```python
from build123d import *

# Parameters (mm, degrees)
SKETCH1_W                      = 60
SKETCH1_H                      = 430.5
BASE_FLANGE1_DEPTH             = 4
EDGE_FLANGE1_STRIP_W           = 18
EDGE_FLANGE1_STRIP_H           = 4
EDGE_FLANGE1_STRIP_CUT_DEPTH   = 430.5
EDGE_FLANGE1_DEPTH             = 430.5
EDGE_FLANGE2_STRIP_W           = 18
EDGE_FLANGE2_STRIP_H           = 4
EDGE_FLANGE2_STRIP_CUT_DEPTH   = 55
EDGE_FLANGE2_STRIP_2_W         = 18
EDGE_FLANGE2_STRIP_2_H         = 4
EDGE_FLANGE2_STRIP_CUT_2_DEPTH = 55
EDGE_FLANGE2_STRIP_3_W         = 18
EDGE_FLANGE2_STRIP_3_H         = 4
EDGE_FLANGE2_STRIP_CUT_3_DEPTH = 55
EDGE_FLANGE2_STRIP_4_W         = 18
EDGE_FLANGE2_STRIP_4_H         = 4
EDGE_FLANGE2_STRIP_CUT_4_DEPTH = 55
EDGE_FLANGE2_DEPTH             = 55
EDGE_FLANGE2_BEND_DEPTH        = 55
EDGE_FLANGE2_BEND_2_DEPTH      = 55
EDGE_FLANGE2_BEND_3_DEPTH      = 55
SKETCH18_R                     = 4.6
EXTRUDE1_DEPTH                 = 440.643321341


# Sheet-metal steps are written as plain solids
with BuildPart() as part:
    # Sketch1 → Base-Flange1 (new body)
    with BuildSketch(Plane(origin=(0, 0, 0), x_dir=(1, 0, 0), z_dir=(0, 1, 0))):
        Rectangle(SKETCH1_W, SKETCH1_H)
    extrude(amount=BASE_FLANGE1_DEPTH)

    # Edge-Flange1 strip (across the edge) → Edge-Flange1 strip cut (cut)
    with BuildSketch(Plane(origin=(-30, 4, -215.25), x_dir=(1, 0, 0), z_dir=(0, 0, 1))):
        with Locations((-4, -2)):
            Rectangle(EDGE_FLANGE1_STRIP_W, EDGE_FLANGE1_STRIP_H)
    extrude(amount=EDGE_FLANGE1_STRIP_CUT_DEPTH, mode=Mode.SUBTRACT)

    # Edge-Flange1 section (across the edge) → Edge-Flange1 (add)
    with BuildSketch(Plane(origin=(-30, 4, -215.25), x_dir=(1, 0, 0), z_dir=(0, 0, 1))):
        with BuildLine():
            Line((0, 1), (0, 56))
            Line((0, 56), (4, 56))
            Line((4, 56), (4, 1))
            ThreePointArc((4, 1), (4.292893219, 0.292893219), (5, 0))
            Line((5, 0), (5, -4))
            ThreePointArc((5, -4), (1.464466094, -2.535533906), (0, 1))
        make_face()
    extrude(amount=EDGE_FLANGE1_DEPTH)

    # Edge-Flange2 strip (across the edge) → Edge-Flange2 strip cut (cut)
    with BuildSketch(Plane(origin=(-30, 5, 215.25), x_dir=(0, 0, -1), z_dir=(0, 1, 0))):
        with Locations((-4, -2)):
            Rectangle(EDGE_FLANGE2_STRIP_W, EDGE_FLANGE2_STRIP_H)
    extrude(amount=EDGE_FLANGE2_STRIP_CUT_DEPTH, mode=Mode.SUBTRACT)

    # Edge-Flange2 strip 2 (across the edge) → Edge-Flange2 strip cut 2 (cut)
    with BuildSketch(Plane(origin=(30, 0, 215.25), x_dir=(0, 0, -1), z_dir=(-1, 0, 0))):
        with Locations((-4, -2)):
            Rectangle(EDGE_FLANGE2_STRIP_2_W, EDGE_FLANGE2_STRIP_2_H)
    extrude(amount=EDGE_FLANGE2_STRIP_CUT_2_DEPTH, mode=Mode.SUBTRACT)

    # Edge-Flange2 strip 3 (across the edge) → Edge-Flange2 strip cut 3 (cut)
    with BuildSketch(Plane(origin=(-30, 60, -215.25), x_dir=(0, 0, 1), z_dir=(0, -1, 0))):
        with Locations((-4, -2)):
            Rectangle(EDGE_FLANGE2_STRIP_3_W, EDGE_FLANGE2_STRIP_3_H)
    extrude(amount=EDGE_FLANGE2_STRIP_CUT_3_DEPTH, mode=Mode.SUBTRACT)

    # Edge-Flange2 strip 4 (across the edge) → Edge-Flange2 strip cut 4 (cut)
    with BuildSketch(Plane(origin=(-25, 0, -215.25), x_dir=(0, 0, 1), z_dir=(1, 0, 0))):
        with Locations((-4, -2)):
            Rectangle(EDGE_FLANGE2_STRIP_4_W, EDGE_FLANGE2_STRIP_4_H)
    extrude(amount=EDGE_FLANGE2_STRIP_CUT_4_DEPTH, mode=Mode.SUBTRACT)

    # Edge-Flange2 section (across the edge) → Edge-Flange2 (add)
    with BuildSketch(Plane(origin=(-30, 5, 215.25), x_dir=(0, 0, -1), z_dir=(0, 1, 0))):
        with BuildLine():
            Line((0, 1), (0, 36))
            Line((0, 36), (4, 36))
            Line((4, 36), (4, 1))
            ThreePointArc((4, 1), (4.292893219, 0.292893219), (5, 0))
            Line((5, 0), (5, -4))
            ThreePointArc((5, -4), (1.464466094, -2.535533906), (0, 1))
        make_face()
    extrude(amount=EDGE_FLANGE2_DEPTH)

    # Edge-Flange2 section 2 (across the edge) → Edge-Flange2 bend (add)
    with BuildSketch(Plane(origin=(30, 0, 215.25), x_dir=(0, 0, -1), z_dir=(-1, 0, 0))):
        with BuildLine():
            Line((0, 1), (0, 36))
            Line((0, 36), (4, 36))
            Line((4, 36), (4, 1))
            ThreePointArc((4, 1), (4.292893219, 0.292893219), (5, 0))
            Line((5, 0), (5, -4))
            ThreePointArc((5, -4), (1.464466094, -2.535533906), (0, 1))
        make_face()
    extrude(amount=EDGE_FLANGE2_BEND_DEPTH)

    # Edge-Flange2 section 3 (across the edge) → Edge-Flange2 bend 2 (add)
    with BuildSketch(Plane(origin=(-30, 60, -215.25), x_dir=(0, 0, 1), z_dir=(0, -1, 0))):
        with BuildLine():
            Line((0, 1), (0, 36))
            Line((0, 36), (4, 36))
            Line((4, 36), (4, 1))
            ThreePointArc((4, 1), (4.292893219, 0.292893219), (5, 0))
            Line((5, 0), (5, -4))
            ThreePointArc((5, -4), (1.464466094, -2.535533906), (0, 1))
        make_face()
    extrude(amount=EDGE_FLANGE2_BEND_2_DEPTH)

    # Edge-Flange2 section 4 (across the edge) → Edge-Flange2 bend 3 (add)
    with BuildSketch(Plane(origin=(-25, 0, -215.25), x_dir=(0, 0, 1), z_dir=(1, 0, 0))):
        with BuildLine():
            Line((0, 1), (0, 36))
            Line((0, 36), (4, 36))
            Line((4, 36), (4, 1))
            ThreePointArc((4, 1), (4.292893219, 0.292893219), (5, 0))
            Line((5, 0), (5, -4))
            ThreePointArc((5, -4), (1.464466094, -2.535533906), (0, 1))
        make_face()
    extrude(amount=EDGE_FLANGE2_BEND_3_DEPTH)

    # Sketch18 → Extrude1 (cut, through all)
    with BuildSketch(Plane.XY.offset(215.25)):
        with Locations((-46, 47.5)):
            Circle(SKETCH18_R)
        with Locations((-46, 17.5)):
            Circle(SKETCH18_R)
        with Locations((-12.5, -16)):
            Circle(SKETCH18_R)
        with Locations((17.5, -16)):
            Circle(SKETCH18_R)
    extrude(amount=-EXTRUDE1_DEPTH, mode=Mode.SUBTRACT)


solid = part.part
```
Can you work these out from the model? Positions are in its coordinate system, mm. A direction names the side the tool comes from. Round coordinates to 2 decimals unless told otherwise and drop trailing zeros. Order: outer loops, then holes, each group sorted by start corner. A loop starts at its lowest first (then second) coordinate and runs counter-clockwise, first axis right, second up. Notation, with made-up numbers: (54, -26.75) -> (108, -26.75) arc R10 cw to (108, -7.75) -> close; hole circle Ø7 at (77, -9). An arc over 180 degrees is marked (long way). Return JSON: item names as keys, results as strings. Group by question number.
1. If we section it at B-B, the plane y = -28.5: Write out the boundary of the cut face in (x, z).
2. If we section it at C-C, the plane y = 47.5: Write out the boundary of the cut face in (x, z), then the cut area to 3 significant figures.
3. We'd pull the mould along Y, two halves only. Please class faces 1 (the face through (-41.75, 45.74, 213.28)), 2 (the face through (2, 4, -3)), 3 (the face through (-30, 32, -3)): released by +Y, released by -Y, zero draft, split by the parting line, or undercut.
4. I need wall thicknesses on line 1 (Y direction, x = -46, z = 212.25); line 2 (Z direction, x = -41.5, y = 52.5); line 3 (Y direction, x = 22, z = -73). Which ranges of each line are inside material? Lowest first, please. Write a range as [from, to].
5. Will these pins go through, and if not, where does the flat tip stop? pin 1 (1.5 mm diameter, centred on x = -9, z = -151, fed in from -Y); pin 2 (12 mm diameter, centred on x = 11.5, y = 0.5, fed in from +Z); pin 3 (1 mm diameter, centred on x = -23.5, z = 167.5, fed in from +Y); pin 4 (6 mm diameter, centred on y = 11, z = -40.5, fed in from -X).
6. If we section it at A-A, the plane x = -46: Write out the boundary of the cut face in (y, z).
7. Which directions (+Z, -Z, +X, -X, +Y, -Y) give clear straight access to the entire face, cutting with the end or side of a thin tool? Please do faces 4 (the face through (-49, 33, -211.25)), 5 (the face through (2, 0, -3)), 6 (the face through (-26, 33, -3)).
8. If we section it at D-D, the plane x = -12.5: Write out the boundary of the cut face in (y, z).
Output values:
{
 "1": {"outline": "(-25, -215.25) -> (30, -215.25) -> (30, -211.25) -> (-25, -211.25) -> close; (-25, 211.25) -> (30, 211.25) -> (30, 215.25) -> (-25, 215.25) -> close"},
 "2": {"outline": "(-66, -215.25) -> (-50.6, -215.25) -> (-50.6, -211.25) -> (-66, -211.25) -> close; (-66, 211.25) -> (-50.6, 211.25) -> (-50.6, 215.25) -> (-66, 215.25) -> close; (-41.4, -215.25) -> (-31, -215.25) arc R5 ccw to (-26, -210.25) -> (-26, 210.25) arc R5 ccw to (-31, 215.25) -> (-41.4, 215.25) -> (-41.4, 211.25) -> (-31, 211.25) arc R1 cw to (-30, 210.25) -> (-30, -210.25) arc R1 cw to (-31, -211.25) -> (-41.4, -211.25) -> close", "area": "1,930 mm²"},
 "3": {"face 1": "undercut", "face 2": "released by +Y", "face 3": "zero draft"},
 "4": {"line 1": "[5, 12.9], [22.1, 42.9], [52.1, 60]", "line 2": "[-215.25, -211.25], [211.25, 215.25]", "line 3": "[0, 4]"},
 "5": {"pin 1": "y = 0", "pin 2": "z = 215.25", "pin 3": "y = 4", "pin 4": "x = -30"},
 "6": {"outline": "(5, -215.25) -> (12.9, -215.25) -> (12.9, -211.25) -> (5, -211.25) -> close; (5, 211.25) -> (12.9, 211.25) -> (12.9, 215.25) -> (5, 215.25) -> close; (22.1, -215.25) -> (42.9, -215.25) -> (42.9, -211.25) -> (22.1, -211.25) -> close; (22.1, 211.25) -> (42.9, 211.25) -> (42.9, 215.25) -> (22.1, 215.25) -> close; (52.1, -215.25) -> (60, -215.25) -> (60, -211.25) -> (52.1, -211.25) -> close; (52.1, 211.25) -> (60, 211.25) -> (60, 215.25) -> (52.1, 215.25) -> close"},
 "7": {"face 4": "-X, +Y, -Y", "face 5": "+X, -X, -Y", "face 6": "+Z, -Z, +X, +Y"},
 "8": {"outline": "(-36, -215.25) -> (-20.6, -215.25) -> (-20.6, -211.25) -> (-36, -211.25) -> close; (-36, 211.25) -> (-20.6, 211.25) -> (-20.6, 215.25) -> (-36, 215.25) -> close; (-11.4, -215.25) -> (-1, -215.25) arc R5 ccw to (4, -210.25) -> (4, 210.25) arc R5 ccw to (-1, 215.25) -> (-11.4, 215.25) -> (-11.4, 211.25) -> (-1, 211.25) arc R1 cw to (0, 210.25) -> (0, -210.25) arc R1 cw to (-1, -211.25) -> (-11.4, -211.25) -> close"}
}
